Verification items for the finished model (mm, model axes). Face numbers are marked on the shaded views. Round coordinates to 2 decimals unless told otherwise and drop trailing zeros. Write each loop counter-clockwise with the first axis right and the second up, starting at its lowest first coordinate (ties: lowest second). Pieces come first, ordered by that corner, then holes. Notation, with made-up numbers: (-15.5, -1) - (-6.5, -1) arc R28 cw to (-6.5, 35) - close; hole circle Ø10 at (57.25, 87.25). An arc over 180 degrees is marked (long way). Answer as a JSON object with one key per item and string values.
```python
from build123d import *

# Parameters (mm, degrees)
SKETCH1_R               = 4.5
BOSS_EXTRUDE1_DEPTH     = 1.5
SKETCH2_W               = 1.75
SKETCH2_H               = 22
BOSS_EXTRUDE2_DEPTH     = 12
SKETCH3_W               = 40
SKETCH3_H               = 50
SKETCH3_W_2             = 32
SKETCH3_H_2             = 42
BOSS_EXTRUDE3_DEPTH     = 2.5
CUT_EXTRUDE1_DEPTH      = 45.263416045
CUT_EXTRUDE1_DEPTH_BACK = 45.263416045
SKETCH3_2_W             = 32
SKETCH3_2_H             = 42
FILLET1_R               = 2
FILLET2_R               = 2
FILLET3_R               = 5


with BuildPart() as part:
    # Sketch1 → Boss-Extrude1 (new body)
    with BuildSketch(Plane(origin=(0, 0, 0), x_dir=(1, 0, 0), z_dir=(0, 1, 0))):
        with BuildLine():
            Line((27.5, -25), (-27.5, -25))
            ThreePointArc((-27.5, -25), (-34.5, -18), (-27.5, -11))
            Line((-27.5, -11), (-21.75, -11))
            Line((-21.75, -11), (-21.75, 11))
            Line((-21.75, 11), (-27.5, 11))
            ThreePointArc((-27.5, 11), (-34.5, 18), (-27.5, 25))
            Line((-27.5, 25), (27.5, 25))
            ThreePointArc((27.5, 25), (34.5, 18), (27.5, 11))
            Line((27.5, 11), (21.75, 11))
            Line((21.75, 11), (21.75, -11))
            Line((21.75, -11), (27.5, -11))
            ThreePointArc((27.5, -11), (34.5, -18), (27.5, -25))
        make_face()
        with Locations(Location((27.5, 18, 0), (0, 0, 270))):
            Circle(SKETCH1_R, mode=Mode.SUBTRACT)
        with Locations(Location((-27.5, 18, 0), (0, 0, 270))):
            Circle(SKETCH1_R, mode=Mode.SUBTRACT)
        with Locations(Location((-27.5, -18, 0), (0, 0, 270))):
            Circle(SKETCH1_R, mode=Mode.SUBTRACT)
        with Locations(Location((27.5, -18, 0), (0, 0, 270))):
            Circle(SKETCH1_R, mode=Mode.SUBTRACT)
    extrude(amount=BOSS_EXTRUDE1_DEPTH)

    # Sketch2 → Boss-Extrude2 (add)
    with BuildSketch(Plane(origin=(0, 1.5, 0), x_dir=(1, 0, 0), z_dir=(0, 1, 0))):
        with Locations((20.875, 0)):
            Rectangle(SKETCH2_W, SKETCH2_H)
        with Locations((-20.875, 0)):
            Rectangle(SKETCH2_W, SKETCH2_H)
    extrude(amount=BOSS_EXTRUDE2_DEPTH)

    # Sketch3 → Boss-Extrude3 (add)
    with BuildSketch(Plane(origin=(0, 1.5, 0), x_dir=(1, 0, 0), z_dir=(0, 1, 0))):
        Rectangle(SKETCH3_W, SKETCH3_H)
        Rectangle(SKETCH3_W_2, SKETCH3_H_2, mode=Mode.SUBTRACT)
    extrude(amount=BOSS_EXTRUDE3_DEPTH)

    # Sketch3_2 → Cut-Extrude1 (cut, two sides: drawn at the far end of the back side and taken through both)
    with BuildSketch(Plane(origin=(0, 1.5, 0), x_dir=(1, 0, 0), z_dir=(0, 1, 0)).offset(-CUT_EXTRUDE1_DEPTH_BACK)):
        Rectangle(SKETCH3_2_W, SKETCH3_2_H)
    extrude(amount=CUT_EXTRUDE1_DEPTH + CUT_EXTRUDE1_DEPTH_BACK, mode=Mode.SUBTRACT)

    # Fillet1
    fillet1_edges = [part.edges().sort_by_distance(p)[0] for p in [
        (-20, 2.75, -25),
        (-20, 2.75, 25),
        (20, 2.75, 25),
        (20, 2.75, -25),
    ]]
    fillet(fillet1_edges, radius=FILLET1_R)

    # Fillet2
    fillet2_edges = [part.edges().sort_by_distance(p)[0] for p in [
        (-16, 2, -21),
        (-16, 2, 21),
        (16, 2, 21),
        (16, 2, -21),
    ]]
    fillet(fillet2_edges, radius=FILLET2_R)

    # Fillet3
    fillet3_edges = [part.edges().sort_by_distance(p)[0] for p in [
        (20.875, 13.5, 11),
        (20.875, 13.5, -11),
        (-20.875, 13.5, -11),
        (-20.875, 13.5, 11),
    ]]
    fillet(fillet3_edges, radius=FILLET3_R)


solid = part.part
```
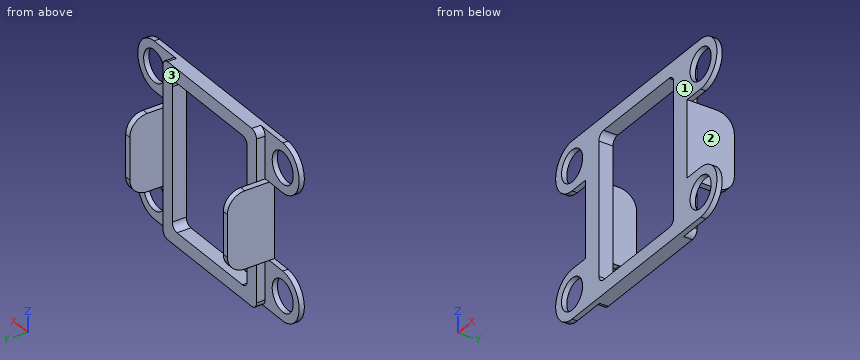
Q1. Section check A-A, the plane z = -18. Record the cut outline in (x, y).
Geometry check:
{"outline": "(-34.5, 0) - (-32, 0) - (-32, 1.5) - (-34.5, 1.5) - close; (-23, 0) - (-16, 0) - (-16, 4) - (-20, 4) - (-20, 1.5) - (-23, 1.5) - close; (16, 0) - (23, 0) - (23, 1.5) - (20, 1.5) - (20, 4) - (16, 4) - close; (32, 0) - (34.5, 0) - (34.5, 1.5) - (32, 1.5) - close"}
Q2. Release check for a two-part mould opening along X. For the marked faces 1, 2 and 3 record: released by +X, released by -X, zero draft, split by the parting line, or undercut.
Geometry check:
{"face 1": "zero draft", "face 2": "released by +X", "face 3": "undercut"}
Q3. Section check B-B, the plane y = 2.5. Record the cut outline in (x, z).
Geometry check:
{"outline": "(-21.75, -11) - (-20, -11) - (-20, -23) arc R2 ccw to (-18, -25) - (18, -25) arc R2 ccw to (20, -23) - (20, -11) - (21.75, -11) - (21.75, 11) - (20, 11) - (20, 23) arc R2 ccw to (18, 25) - (-18, 25) arc R2 ccw to (-20, 23) - (-20, 11) - (-21.75, 11) - close; hole (-16, -19) arc R2 ccw to (-14, -21) - (14, -21) arc R2 ccw to (16, -19) - (16, 19) arc R2 ccw to (14, 21) - (-14, 21) arc R2 ccw to (-16, 19) - close"}
Q4. Material ranges on line 1 along X through (y, z) = (0.95, 18); line 2 along X through (y, z) = (0.5, -1); line 3 along Z through (x, y) = (-3, 3.5), recorded low to high. Write a range as [from, to].
Geometry check:
{"line 1": "x = [-34.5, -32], [-23, -16], [16, 23], [32, 34.5]", "line 2": "x = [-21.75, -16], [16, 21.75]", "line 3": "z = [-25, -21], [21, 25]"}
Q5. Section check C-C, the plane x = -13. Record the cut outline in (y, z), then the cut area to 3 significant figures.
Geometry check:
{"outline": "(0, -25) - (4, -25) - (4, -21) - (0, -21) - close; (0, 21) - (4, 21) - (4, 25) - (0, 25) - close", "area": "32.0 mm2"}
Q6. Gauge pin test, flat ends, axial feed: P1, Ø0.8, axis at y = 3, z = 19, coming from the -X side; P2, Ø11, axis at x = 23, z = -17, coming from the +Y side; P3, Ø1.9, axis at x = -21.5, y = 4, coming from the -Z side. Record the tip position at first contact, or that the pin passes through.
Geometry check:
{"P1": "stops at x = -20", "P2": "stops at y = 4", "P3": "stops at z = -11"}
Q7. Section check D-D, the plane z = 9.5. Record the cut outline in (x, y).
Geometry check:
{"outline": "(-21.75, 0) - (-16, 0) - (-16, 4) - (-20, 4) - (-20, 12.07) - (-21.75, 12.07) - close; (16, 0) - (21.75, 0) - (21.75, 12.07) - (20, 12.07) - (20, 4) - (16, 4) - close"}
